```python
from build123d import *

# Parameters (mm, degrees)
CHAMFER1_SIZE   = 0.25
HEX_2_DEPTH     = 10
THDSCHPAT_COUNT = 8
THDSCHPAT_PITCH = 2.325


with BuildPart() as part:
    # BodySke → BaseBody (revolve)
    with BuildSketch(Plane.XY, mode=Mode.PRIVATE) as basebody_sk:
        with BuildLine():
            Line((0, 0), (0, 18))
            Line((0, 18), (16, 18))
            Line((16, 18), (16, 12.49))
            Line((16, 12.49), (66, 12.49))
            Line((66, 12.49), (66, 9.53))
            ThreePointArc((66, 9.53), (66.404192642, 8.554192642), (67.38, 8.15))
            Line((67.38, 8.15), (72.3, 8.15))
            Line((72.3, 8.15), (74.15, 10))
            Line((74.15, 10), (92.2985, 10))
            Line((92.2985, 10), (93.4, 8.8985))
            Line((93.4, 8.8985), (93.4, 0))
            Line((93.4, 0), (0, 0))
        make_face()
    revolve(basebody_sk.sketch.rotate(Axis((-6.35, 0, 0), (1, 0, 0)), 90), axis=Axis((-6.35, 0, 0), (1, 0, 0)))

    # Chamfer1
    chamfer1_edges = [part.edges().sort_by_distance(p)[0] for p in [
        (0, 0, -18),
    ]]
    chamfer(chamfer1_edges, length=CHAMFER1_SIZE)

    # Sketch2 → PreBroach (revolve, cut)
    with BuildSketch(Plane.XY, mode=Mode.PRIVATE) as prebroach_sk:
        Polygon((0, 6), (10, 6), (13.464101615, 0), (0, 0), align=None)
    revolve(prebroach_sk.sketch.rotate(Axis((0, 0, 0), (1, 0, 0)), 90), axis=Axis((0, 0, 0), (1, 0, 0)), mode=Mode.SUBTRACT)

    # Sketch3 → Hex 2 (cut)
    with BuildSketch(Plane.ZY):
        Polygon((-6, -3.464101615), (-6, 3.464101615), (0, 6.92820323), (6, 3.464101615), (6, -3.464101615), (0, -6.92820323), align=None)
    extrude(amount=-HEX_2_DEPTH, mode=Mode.SUBTRACT)

    # ThdSchSke → ThreadSchematic (revolve, cut)
    with BuildSketch(Plane.XY):
        Polygon((74.8, -8.8985), (72.285204627, -12.49), (72.285204627, -15.6125), (77.314795373, -15.6125), (77.314795373, -12.49), align=None)
    threadschematic = revolve(axis=Axis((-3.175, 0, 0), (1, 0, 0)), mode=Mode.SUBTRACT)

    # ThdSchPat: ThreadSchematic ×8
    with Locations(*[(i * THDSCHPAT_PITCH, 0, 0) for i in range(1, THDSCHPAT_COUNT)]):
        add(threadschematic, mode=Mode.SUBTRACT)


solid = part.part
```
Part model, mm, in its own coordinate system. A direction names the side the tool comes from. Round coordinates to 2 decimals unless told otherwise and drop trailing zeros. Write each loop counter-clockwise with the first axis right and the second up, starting at its lowest first coordinate (ties: lowest second). Pieces come first, ordered by that corner, then holes. Notation, with made-up numbers: (45.5, 40) -> (98.5, 40) arc R26 ccw to (98.5, 65) -> close; hole circle Ø9 at (-6.5, 32.25). An arc over 180 degrees is marked (long way). Return JSON: item names as keys, results as strings. Group by question number.
Q1. Probe L1, parallel to Y at x = 5.5, z = 0; L2, parallel to Z at x = 40.5, y = 0.5; L3, parallel to X at y = 13, z = 10. List the from-to ranges inside material, lowest first. Write a range as [from, to].
Q2. Pin check, flat tips, straight feed: pin 1 (2 mm diameter, centred on x = 66.5, z = -8, fed in from -Y); pin 2 (1.5 mm diameter, centred on y = -8.5, z = -12.5, fed in from +X); pin 3 (2.5 mm diameter, centred on y = 1.5, z = -4, fed in from -X); pin 4 (3.5 mm diameter, centred on y = -3.5, z = 5, fed in from -X). Stop position of each tip, or through.
Q3. Which spindle directions (+Z, -Z, +X, -X, +Y, -Y) get a long thin tool onto all of the face, cutting with end or side? Do faces 1 (the cylindrical face through (92, 0, -10)), 2 (the flat face through (10, -3.2, 5.4)), 3 (the conical face through (82, 2, 9)). Say none if no direction does.
Q4. Saw through at A-A on x = 11. Write the cut outline in (y, z).
Q5. Mould opens along Y. For faces 4 (the flat face through (93.4, 0, 0)), 5 (the flat face through (10, -3.2, -5.4)), 6 (the cylindrical face through (83, 0, -10)) say: pulls with the +Y half, pulls with the -Y half, needs draft (parallel to the pull), parting line crosses it, or undercut.
Answer:
{
 "1": {"L1": "[-18, -6.93], [6.93, 18]", "L2": "[-12.48, 12.48]", "L3": "[0, 16]"},
 "2": {"pin 1": "y = -10.25", "pin 2": "x = 16", "pin 3": "x = 10.28", "pin 4": "x = 0"},
 "3": {"face 1": "+X", "face 2": "-X", "face 3": "none"},
 "4": {"outline": "circle Ø36 at (0, 0); hole circle Ø8.54 at (0, 0)"},
 "5": {"face 4": "needs draft", "face 5": "undercut", "face 6": "parting line crosses it"}
}
